Work out the finished part from the listing and answer in its coordinate system (mm). Give positions to 0.01 mm unless a question says otherwise; leave off trailing zeros. Order: outer loops, then holes, each group sorted by start corner. A loop starts at its lowest first (then second) coordinate and runs counter-clockwise, first axis right, second up.
```python
from build123d import *

# Parameters (mm, degrees)
SZKIC1_W                    = 0.64
SZKIC1_H                    = 0.64
DODANIE_WYCI_GNI_CIE1_DEPTH = 14.2
SFAZOWANIE1_SIZE            = 0.25
SFAZOWANIE2_SIZE            = 0.25


with BuildPart() as part:
    # Szkic1 → Dodanie-wyciągnięcie1 (new body)
    with BuildSketch(Plane(origin=(0, 0, 0), x_dir=(1, 0, 0), z_dir=(0, 1, 0))):
        Rectangle(SZKIC1_W, SZKIC1_H)
    extrude(amount=DODANIE_WYCI_GNI_CIE1_DEPTH)

    # Sfazowanie1
    sfazowanie1_edges = [part.edges().sort_by_distance(p)[0] for p in [
        (0.32, 14.2, 0),
        (0, 14.2, -0.32),
        (-0.32, 14.2, 0),
        (0, 14.2, 0.32),
    ]]
    chamfer(sfazowanie1_edges, length=SFAZOWANIE1_SIZE)

    # Sfazowanie2
    sfazowanie2_edges = [part.edges().sort_by_distance(p)[0] for p in [
        (0, 0, -0.32),
        (0.32, 0, 0),
        (0, 0, 0.32),
        (-0.32, 0, 0),
    ]]
    chamfer(sfazowanie2_edges, length=SFAZOWANIE2_SIZE)


solid = part.part
```
1. The part is cut by section B-B (z = -0.2). Write down the section's boundary in (x, y).
Findings below:
outline: (-0.32, 0.25) - (-0.2, 0.13) - (0.2, 0.13) - (0.32, 0.25) - (0.32, 13.95) - (0.2, 14.07) - (-0.2, 14.07) - (-0.32, 13.95) - close
2. Straight lines are drawn through the part: probe 1 along Y at (x, z) = (-0.2, 0); probe 2 along Y at (x, z) = (0.1, 0.25). For each, find the intervals that lie inside material, in ascending order.
Findings below:
probe 1: y = 0.13 to 14.07
probe 2: y = 0.18 to 14.02
3. The part is cut by section A-A (x = 0.2). Write down the section's boundary in (y, z), then the cut area to 3 significant figures.
Findings below:
outline: (0.13, -0.2) - (0.25, -0.32) - (13.95, -0.32) - (14.07, -0.2) - (14.07, 0.2) - (13.95, 0.32) - (0.25, 0.32) - (0.13, 0.2) - close
area: 8.89 mm2
